Autodesk Inventor part; units mm, degrees
ref_plane "YZ Plane" through (0, 0, 0) normal (1, 0, 0) x (0, 1, 0)
ref_plane "XZ Plane" through (0, 0, 0) normal (0, 1, 0) x (-1, 0, 0)
ref_plane "XY Plane" through (0, 0, 0) normal (0, 0, 1) x (1, 0, 0)
sketch "Sketch1" plane through (0, 0, 0) normal (0, 0, 1) x (1, 0, 0)
  line L0 (0, 0) -> (67.31, 0)
  line L1 (67.31, 0) -> (67.31, 52)
  line L2 (67.31, 52) -> (0, 52)
  line L3 (0, 52) -> (0, 0)
  line L4 (4, 8) -> (63.31, 8)
  line L5 (63.31, 8) -> (63.31, 32)
  line L6 (63.31, 32) -> (4, 32)
  line L7 (4, 32) -> (4, 8)
  dimension "d0" = 67.31
  dimension "d1" = 52
  dimension "d2" = 59.31
  dimension "d4" = 4
  dimension "d5" = 8
  dimension "d19" = 20
extrude "Extrusion1" add sketch "Sketch1" along normal blind 2
sketch "Sketch2" plane through (0, 0, 2) normal (0, 0, 1) x (1, 0, 0)
  line L0 (0, 0) -> (67.31, 0)
  line L1 (4, 0) -> (4, 39.8865)
  line L2 (0, 52) -> (0, 0)
  line L3 (0, 48) -> (67.31, 48)
  line L4 (63.31, 39.878) -> (63.31, 0)
  line L5 (0, 4) -> (67.31, 4)
  line L6 (67.31, 52) -> (0, 52)
  line L7 (67.31, 0) -> (67.31, 52)
  point P0 (4, 48)
  point P1 (4, 4)
  point P2 (63.31, 4)
  point P3 (63.31, 48)
  dimension "d8" = 4
  dimension "d9" = 4
  dimension "d10" = 4
  dimension "d11" = 4
hole "Hole1" at (4, 48, 2) at (4, 4, 2) at (63.31, 4, 2) at (63.31, 48, 2) direction (0, 0, -1) diameter 4.5 end through all
fillet "Fillet1" radius 2 4 edges at (0, 52, 1) (0, 0, 1) (67.31, 0, 1) (67.31, 52, 1)
fillet "Fillet2" radius 2 4 edges at (63.31, 8, 1) (63.31, 32, 1) (4, 32, 1) (4, 8, 1)
properties part number "cosmic-watch-endplate"
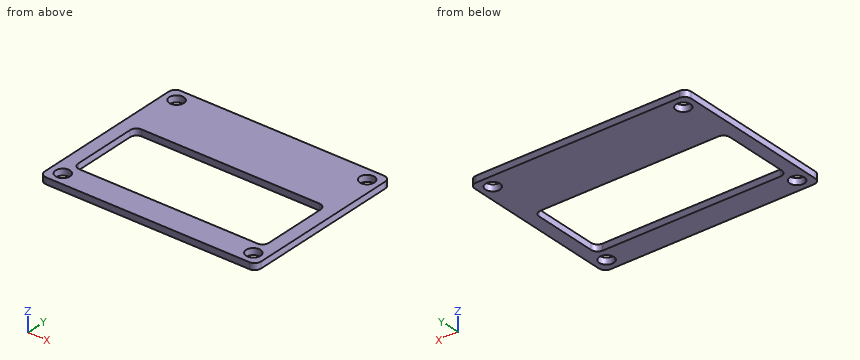
Here's how the part is built. I have some questions about the finished solid (model axes, mm). Give positions to 0.01 mm unless a question says otherwise; leave off trailing zeros. Loops run counter-clockwise (first coordinate to the right, second up) from the corner with the lowest first, then second, coordinate; pieces in that order, holes last. Notation, with made-up numbers: M 58.5,-19 L 68.5,-19 A17 cw 68.5,-7 Z; hole C 50.25,26.25 d5. An arc over 180 degrees is marked long. Use one line per item in the form item = value. Start each with the question number.
Q1. I need wall thicknesses on line 1 along X through (y, z) = (4, 0.5); line 2 along X through (y, z) = (5, 1.4); line 3 along Y through (x, z) = (31, 0.95). Which ranges of each line are inside material? Lowest first, please.
Q2. Will this pin go through, and if not, where does the flat tip stop? pin 1 Ø7 at (x, y) = (4, 4) entering from +Z.
Q3. If we section it at D-D (z = 0.5): Write out the boundary of the cut face in (x, y).
Q4. If we section it at A-A (y = 48): Write out the boundary of the cut face in (x, z), then the cut area to 3 significant figures.
Q5. If we section it at C-C (x = 53.5): Write out the boundary of the cut face in (y, z), then the cut area to 3 significant figures.
Q6. If we section it at B-B (y = 12): Write out the boundary of the cut face in (x, z), then the cut area to 3 significant figures.
Taken from the geometry:
q1.line_1 = 0 to 1.75, 6.25 to 61.06, 65.56 to 67.31
q1.line_2 = 0 to 1.98, 6.02 to 61.29, 65.33 to 67.31
q1.line_3 = 0 to 8, 32 to 52
q2.pin_1 = 2
q3.outline = M 0,2 A2 ccw 2,0 L 65.31,0 A2 ccw 67.31,2 L 67.31,50 A2 ccw 65.31,52 L 2,52 A2 ccw 0,50 Z; hole C 4,4 d4.5; hole C 4,48 d4.5; hole M 4,10 A2 ccw 6,8 L 61.31,8 A2 ccw 63.31,10 L 63.31,30 A2 ccw 61.31,32 L 6,32 A2 ccw 4,30 Z; hole C 63.31,4 d4.5; hole C 63.31,48 d4.5
q4.outline = M 0,0 L 1.75,0 L 1.75,2 L 0,2 Z; M 6.25,0 L 61.06,0 L 61.06,2 L 6.25,2 Z; M 65.56,0 L 67.31,0 L 67.31,2 L 65.56,2 Z
q4.area = 117 mm^2
q5.outline = M 0,0 L 8,0 L 8,2 L 0,2 Z; M 32,0 L 52,0 L 52,2 L 32,2 Z
q5.area = 56.0 mm^2
q6.outline = M 0,0 L 4,0 L 4,2 L 0,2 Z; M 63.31,0 L 67.31,0 L 67.31,2 L 63.31,2 Z
q6.area = 16.0 mm^2
